Could you check a few things on this model? Use its own coordinates, in mm. A direction names the side the tool comes from. Coordinates: 2 decimals unless noted, no trailing zeros. Write each loop counter-clockwise with the first axis right and the second up, starting at its lowest first coordinate (ties: lowest second). Pieces come first, ordered by that corner, then holes.
```python
from build123d import *

# Parameters (mm, degrees)
ESQUISSE2_W             = 64.9
ESQUISSE2_H             = 84.149666381
ESQUISSE2_R             = 1.45
ESQUISSE2_W_2           = 44.9
ESQUISSE2_H_2           = 64.15
BOSS_EXTRU_3_DEPTH      = 13
ESQUISSE6_W             = 44.9
ESQUISSE6_H             = 64.15
BOSS_EXTRU_4_DEPTH      = 3
ESQUISSE8_W             = 20
ESQUISSE8_H             = 9
ENL_V_MAT_EXTRU_2_DEPTH = 10
CONG_1_R                = 1
CONG_2_R                = 1
CONG_3_R                = 1
CONG_4_R                = 1


with BuildPart() as part:
    # Esquisse2 → Boss.-Extru.3 (new body)
    with BuildSketch(Plane.XY):
        with Locations((-9.785413718, 8.985039615)):
            Rectangle(ESQUISSE2_W, ESQUISSE2_H)
        with Locations(Location((17.664586282, 46.059872806, 0), (0, 0, 180))):
            Circle(ESQUISSE2_R, mode=Mode.SUBTRACT)
        with Locations(Location((-37.235413718, 46.059872806, 0), (0, 0, 180))):
            Circle(ESQUISSE2_R, mode=Mode.SUBTRACT)
        with Locations(Location((-37.235413718, -28.089793575, 0), (0, 0, 180))):
            Circle(ESQUISSE2_R, mode=Mode.SUBTRACT)
        with Locations(Location((17.664586282, -28.089793575, 0), (0, 0, 180))):
            Circle(ESQUISSE2_R, mode=Mode.SUBTRACT)
        with Locations((-9.785413718, 8.985206425)):
            Rectangle(ESQUISSE2_W_2, ESQUISSE2_H_2, mode=Mode.SUBTRACT)
    extrude(amount=BOSS_EXTRU_3_DEPTH)

    # Esquisse6 → Boss.-Extru.4 (add)
    with BuildSketch(Plane.XY):
        with Locations((-9.785413718, 8.985206425)):
            Rectangle(ESQUISSE6_W, ESQUISSE6_H)
    extrude(amount=BOSS_EXTRU_4_DEPTH)

    # Esquisse8 → Enlèv. mat.-Extru.2 (cut)
    with BuildSketch(Plane.XZ.offset(-41.060206425)):
        with Locations((-9.785413718, 8.5)):
            Rectangle(ESQUISSE8_W, ESQUISSE8_H)
    extrude(amount=-ENL_V_MAT_EXTRU_2_DEPTH, mode=Mode.SUBTRACT)

    # Congé1
    cong_1_edges = [part.edges().sort_by_distance(p)[0] for p in [
        (-42.235413718, 51.059872806, 6.5),
    ]]
    fillet(cong_1_edges, radius=CONG_1_R)

    # Congé2
    cong_2_edges = [part.edges().sort_by_distance(p)[0] for p in [
        (-42.235413718, -33.089793575, 6.5),
    ]]
    fillet(cong_2_edges, radius=CONG_2_R)

    # Congé3
    cong_3_edges = [part.edges().sort_by_distance(p)[0] for p in [
        (22.664586282, -33.089793575, 6.5),
    ]]
    fillet(cong_3_edges, radius=CONG_3_R)

    # Congé4
    cong_4_edges = [part.edges().sort_by_distance(p)[0] for p in [
        (22.664586282, 51.059872806, 6.5),
    ]]
    fillet(cong_4_edges, radius=CONG_4_R)


solid = part.part
```
1. I want a section at C-C on x = -37. Please give me the cut outline in (y, z).
Verdict:
outline: (-33.09, 0) - (-29.52, 0) - (-29.52, 13) - (-33.09, 13) - close; (-26.66, 0) - (44.63, 0) - (44.63, 13) - (-26.66, 13) - close; (47.49, 0) - (51.06, 0) - (51.06, 13) - (47.49, 13) - close
2. If we mould it in two halves opening along Y, with no side actions, what happens to faces 1 (the face through (-10, 10, 0)), 2 (the face through (-10.2, 51.06, 3.5)), 3 (the face through (-10, -33.09, 6)), 4 (the face through (12.665, 9, 8))? For each: pulls with the +Y half, pulls with the -Y half, needs draft (parallel to the pull), parting line crosses it, or undercut.
Verdict:
face 1: needs draft
face 2: pulls with the +Y half
face 3: pulls with the -Y half
face 4: undercut
3. Please list where these lines run through material, in increasing order: line 1 along X through (y, z) = (-1, 3.5); line 2 along Y through (x, z) = (-26.5, 5.5); line 3 along Y through (x, z) = (-37.5, 3.5).
Verdict:
line 1: x = -42.24 to -32.24, 12.66 to 22.66
line 2: y = -33.09 to -23.09, 41.06 to 51.06
line 3: y = -33.09 to -29.52, -26.66 to 44.63, 47.49 to 51.06
4. I want a section at B-B on y = -10.5. Please give me the cut outline in (x, z), plus the area to 3 significant figures.
Verdict:
outline: (-42.24, 0) - (22.66, 0) - (22.66, 13) - (12.66, 13) - (12.66, 3) - (-32.24, 3) - (-32.24, 13) - (-42.24, 13) - close
area: 395 mm2
5. I want a section at D-D on z = 7.5. Please give me the cut outline in (x, y).
Verdict:
outline: (-42.24, -32.09) arc R1 ccw to (-41.24, -33.09) - (21.66, -33.09) arc R1 ccw to (22.66, -32.09) - (22.66, 50.06) arc R1 ccw to (21.66, 51.06) - (0.21, 51.06) - (0.21, 41.06) - (12.66, 41.06) - (12.66, -23.09) - (-32.24, -23.09) - (-32.24, 41.06) - (-19.79, 41.06) - (-19.79, 51.06) - (-41.24, 51.06) arc R1 ccw to (-42.24, 50.06) - close; hole circle Ø2.9 at (-37.24, -28.09); hole circle Ø2.9 at (-37.24, 46.06); hole circle Ø2.9 at (17.66, -28.09); hole circle Ø2.9 at (17.66, 46.06)
6. On a 3-axis mill with a long thin cutter (end or side, diameter ignored), from which of +Z, -Z, +X, -X, +Y, -Y can I reach the whole of each face in a straight line? I mean faces 5 (the face through (-19.785, 46, 8)), 6 (the face through (-10, 9, 3)), 7 (the face through (17.979, -26.674, 6.409)). Say none if no direction works.
Verdict:
face 5: +Z, +Y
face 6: +Z
face 7: +Z, -Z
7. For pin 1 (3 mm diameter, centred on x = -14, y = 46.5, fed in from +Z); pin 2 (2.5 mm diameter, centred on x = -37.24, y = -28.09, fed in from +Z); pin 3 (1.5 mm diameter, centred on x = -6.5, y = -13.5, fed in from +Z); pin 4 (4 mm diameter, centred on x = -37.24, y = 46.06, fed in from +Z), each with a flat end and sliding along its axis, tell me the tip position at first contact or that it passes through.
Verdict:
pin 1: stops at z = 4
pin 2: passes through
pin 3: stops at z = 3
pin 4: stops at z = 13
8. I want a section at A-A on x = 11. Please give me the cut outline in (y, z), plus the area to 3 significant figures.
Verdict:
outline: (-33.09, 0) - (51.06, 0) - (51.06, 13) - (41.06, 13) - (41.06, 3) - (-23.09, 3) - (-23.09, 13) - (-33.09, 13) - close
area: 452 mm2
